from build123d import *

# Parameters (mm, degrees)
F0_W            = 219
F0_H            = 225
F1_DEPTH        = 25
F3_DEPTH        = 95
F4_R            = 37.5
F5_DEPTH        = 10
F5_DEPTH_BACK   = 127
F6_R            = 40
F7_DEPTH        = 10
F7_DEPTH_BACK   = 127
F8_W            = 60
F8_H            = 60
F9_DEPTH        = 10
F10_R           = 10
F12_DEPTH       = 20
F14_D           = 15
F14_CBORE_D     = 30
F14_CBORE_DEPTH = 10
F15_R           = 10
F16_R           = 19.5
F17_DEPTH       = 229.001
F18_R           = 19.5
F19_DEPTH       = 235.001
F20_SIZE        = 2
F21_R           = 10


with BuildPart() as f1:
    # F0 (on Top) → F1 (new body)
    with BuildSketch(Plane.XY):
        Rectangle(F0_W, F0_H)
    extrude(amount=F1_DEPTH)

    # F2 (on face) → F3 (join)
    with BuildSketch(Plane.XY.offset(25)):
        with BuildLine():
            Line((-29.5, 63.5), (-109.5, 63.5))
            Line((-109.5, 63.5), (-109.5, 48.5))
            Line((-109.5, 48.5), (-43.571649, 48.5))
            ThreePointArc((-43.571649, 48.5), (-12.195597, -15.195597), (51.5, -46.571649))
            Line((51.5, -46.571649), (51.5, -112.5))
            Line((51.5, -112.5), (66.5, -112.5))
            Line((66.5, -112.5), (66.5, -32.5))
            ThreePointArc((66.5, -32.5), (-1.588995, -4.588995), (-29.5, 63.5))
        make_face()
    extrude(amount=F3_DEPTH)

    # F4 (on face) → F5 (join, two sides)
    with BuildSketch(Plane(origin=(-109.5, 0, 0), x_dir=(0, -1, 0), z_dir=(-1, 0, 0))) as f5_sk:
        with Locations((-56, 120)):
            Circle(F4_R)
    extrude(amount=F5_DEPTH)
    extrude(f5_sk.sketch, amount=-F5_DEPTH_BACK)

    # F6 (on face) → F7 (join, two sides)
    with BuildSketch(Plane.XZ.offset(112.5)) as f7_sk:
        with Locations((59, 120)):
            Circle(F6_R)
    extrude(amount=F7_DEPTH)
    extrude(f7_sk.sketch, amount=-F7_DEPTH_BACK)

    # F8 (on face) → F9 (join)
    with BuildSketch(Plane.XY.offset(25)):
        with Locations((-79.5, -82.5)):
            Rectangle(F8_W, F8_H)
    extrude(amount=F9_DEPTH)

    # F10
    f10_edges = [f1.edges().sort_by_distance(p)[0] for p in [
        (-49.5, -52.5, 30),
    ]]
    fillet(f10_edges, radius=F10_R)

    # F11 (on face) → F12 (cut)
    with BuildSketch(Plane.XY.offset(25)):
        with BuildLine():
            ThreePointArc((42.5, -54.205123), (-18.559558, -21.559558), (-51.205123, 39.5))
            Line((-51.205123, 39.5), (-100.5, 39.5))
            Line((-100.5, 39.5), (-100.5, -43.5))
            Line((-100.5, -43.5), (-59.5, -43.5))
            ThreePointArc((-59.5, -43.5), (-46.064971, -49.064971), (-40.5, -62.5))
            Line((-40.5, -62.5), (-40.5, -103.5))
            Line((-40.5, -103.5), (42.5, -103.5))
            Line((42.5, -103.5), (42.5, -54.205123))
        make_face()
    extrude(amount=-F12_DEPTH, mode=Mode.SUBTRACT)

    # F14 (through all)
    with Locations(Plane.XY.offset(35)):
        with Locations((-79.5, -82.5)):
            CounterBoreHole(F14_D / 2, F14_CBORE_D / 2, F14_CBORE_DEPTH)

    # F15
    f15_edges = [f1.edges().sort_by_distance(p)[0] for p in [
        (42.5, -54.205123, 15),
        (-51.205123, 39.5, 15),
        (42.5, -103.5, 15),
        (-40.5, -103.5, 15),
        (-100.5, 39.5, 15),
        (-100.5, -43.5, 15),
    ]]
    fillet(f15_edges, radius=F15_R)

    # F16 (on face) → F17 (cut, through all)
    with BuildSketch(Plane(origin=(-119.5, 0, 0), x_dir=(0, -1, 0), z_dir=(-1, 0, 0))):
        with Locations((-56, 120)):
            Circle(F16_R)
    extrude(amount=-F17_DEPTH, mode=Mode.SUBTRACT)

    # F18 (on face) → F19 (cut, through all)
    with BuildSketch(Plane.XZ.offset(122.5)):
        with Locations((59, 120)):
            Circle(F18_R)
    extrude(amount=-F19_DEPTH, mode=Mode.SUBTRACT)

    # F20
    f20_edges = [f1.edges().sort_by_distance(p)[0] for p in [
        (-119.5, 75.5, 120),
        (39.5, -122.5, 120),
        (39.5, 14.5, 120),
        (17.5, 75.5, 120),
    ]]
    chamfer(f20_edges, length=F20_SIZE)

    # F21
    f21_edges = [f1.edges().sort_by_distance(p)[0] for p in [
        (-109.5, -112.5, 17.5),
        (109.5, -112.5, 12.5),
        (109.5, 112.5, 12.5),
        (-109.5, 112.5, 12.5),
    ]]
    fillet(f21_edges, radius=F21_R)


solid = f1.part
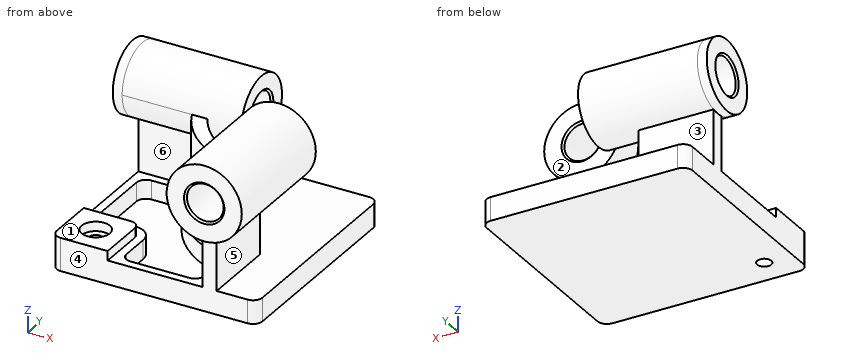
Can you work these out from the model? Positions are in its coordinate system, mm. Face numbers are marked on the shaded views. A direction names the side the tool comes from. Round coordinates to 2 decimals unless told otherwise and drop trailing zeros. Write each loop counter-clockwise with the first axis right and the second up, starting at its lowest first coordinate (ties: lowest second). Pieces come first, ordered by that corner, then holes. Notation, with made-up numbers: (45, -9.5) -> (75, -9.5) arc R29 cw to (75, 19.5) -> close; hole circle Ø11 at (12.25, 75). An arc over 180 degrees is marked (long way). One line per question, with ' | ' between items. Start each with the question number.
1) Suppose I cut it at A-A on x = -79.5. Write out the boundary of the cut face in (y, z), then the cut area to 3 significant figures.
2) I'm going to push flat-ended pins straight in: P1, Ø5, axis at x = -70.5, z = 111, coming from the -Y side; P2, Ø5, axis at y = -90, z = 29, coming from the +X side; P3, Ø12, axis at x = -79.5, y = -82.5, coming from the -Z side; P4, Ø1.5, axis at x = 26, z = 33.5, coming from the -Y side. Where does each tip first touch, or does it pass through?
3) Suppose I cut it at C-C on z = 42. Write out the boundary of the cut face in (x, y), then the cut area to 3 significant figures.
4) Suppose I cut it at D-D on y = 56. Write out the boundary of the cut face in (x, z), then the cut area to 3 significant figures.
5) I need wall thicknesses on line 1 (X direction, y = -82, z = 9); line 2 (Y direction, x = -79, z = 8); line 3 (X direction, y = -82, z = 31). Which ranges of each line are inside material? Lowest first, please. Write a range as [from, to].
6) If we mould it in two halves opening along Z, with no side actions, what happens to the marked faces 1, 2 and 3? For each: released by +Z, released by -Z, zero draft, split by the parting line, or undercut.
7) On a 3-axis mill with a long thin cutter (end or side, diameter ignored), from which of +Z, -Z, +X, -X, +Y, -Y can I reach the whole of each face in a straight line? I mean the marked faces 4, 5 and 6. Say none if no direction works.
8) Suppose I cut it at B-B on y = -82.5. Write out the boundary of the cut face in (x, z), then the cut area to 3 significant figures.
Return value:
1) outline: (-112.5, 0) -> (-90, 0) -> (-90, 25) -> (-97.5, 25) -> (-97.5, 35) -> (-112.5, 35) -> close; (-75, 0) -> (112.5, 0) -> (112.5, 25) -> (63.5, 25) -> (63.5, 83.26) arc R37.5 ccw (long way) to (48.5, 83.26) -> (48.5, 25) -> (39.5, 25) -> (39.5, 5) -> (-43.5, 5) -> (-43.5, 25) -> (-52.5, 25) -> (-52.5, 35) -> (-67.5, 35) -> (-67.5, 25) -> (-75, 25) -> close; hole circle Ø39 at (56, 120) | area: 7,980 mm2
2) P1: stops at y = 19.07 | P2: stops at x = 66.5 | P3: passes through | P4: stops at y = -40.36
3) outline: (-109.5, 48.5) -> (-43.57, 48.5) arc R110.3 ccw to (51.5, -46.57) -> (51.5, -112.5) -> (66.5, -112.5) -> (66.5, -32.5) arc R95.3 cw to (-29.5, 63.5) -> (-109.5, 63.5) -> close | area: 4,400 mm2
4) outline: (-119.5, 82.5) -> (-109.5, 82.5) -> (-109.5, 0) -> (109.5, 0) -> (109.5, 25) -> (-29.26, 25) -> (-29.26, 82.5) -> (17.5, 82.5) -> (17.5, 98.5) -> (15.5, 100.5) -> (-117.5, 100.5) -> (-119.5, 98.5) -> close; (-119.5, 141.5) -> (-117.5, 139.5) -> (15.5, 139.5) -> (17.5, 141.5) -> (17.5, 157.5) -> (-119.5, 157.5) -> close | area: 15,000 mm2
5) line 1: x = [-109.5, -86.98], [-72.02, -40.5], [42.5, 109.5] | line 2: y = [-112.5, -89.98], [-75.02, -43.5], [39.5, 112.5] | line 3: x = [-109.5, -94.49], [-64.51, -49.5], [51.5, 66.5]
6) face 1: released by +Z | face 2: zero draft | face 3: undercut
7) face 4: -Z, +X, -X, -Y | face 5: +X, +Y, -Y | face 6: -X
8) outline: (-109.5, 0) -> (-87, 0) -> (-87, 25) -> (-94.5, 25) -> (-94.5, 35) -> (-109.5, 35) -> close; (-72, 0) -> (109.5, 0) -> (109.5, 25) -> (66.5, 25) -> (66.5, 80.71) arc R40 ccw (long way) to (51.5, 80.71) -> (51.5, 25) -> (42.5, 25) -> (42.5, 5) -> (-40.5, 5) -> (-40.5, 25) -> (-49.5, 25) -> (-49.5, 35) -> (-64.5, 35) -> (-64.5, 25) -> (-72, 25) -> close; hole circle Ø39 at (59, 120) | area: 8,400 mm2
